Here's the drawing with two shaded views (mm, measured from the low corner). I have some questions. Round coordinates to 2 decimals unless told otherwise and drop trailing zeros. Order: outer loops, then holes, each group sorted by start corner. A loop starts at its lowest first (then second) coordinate and runs counter-clockwise, first axis right, second up.
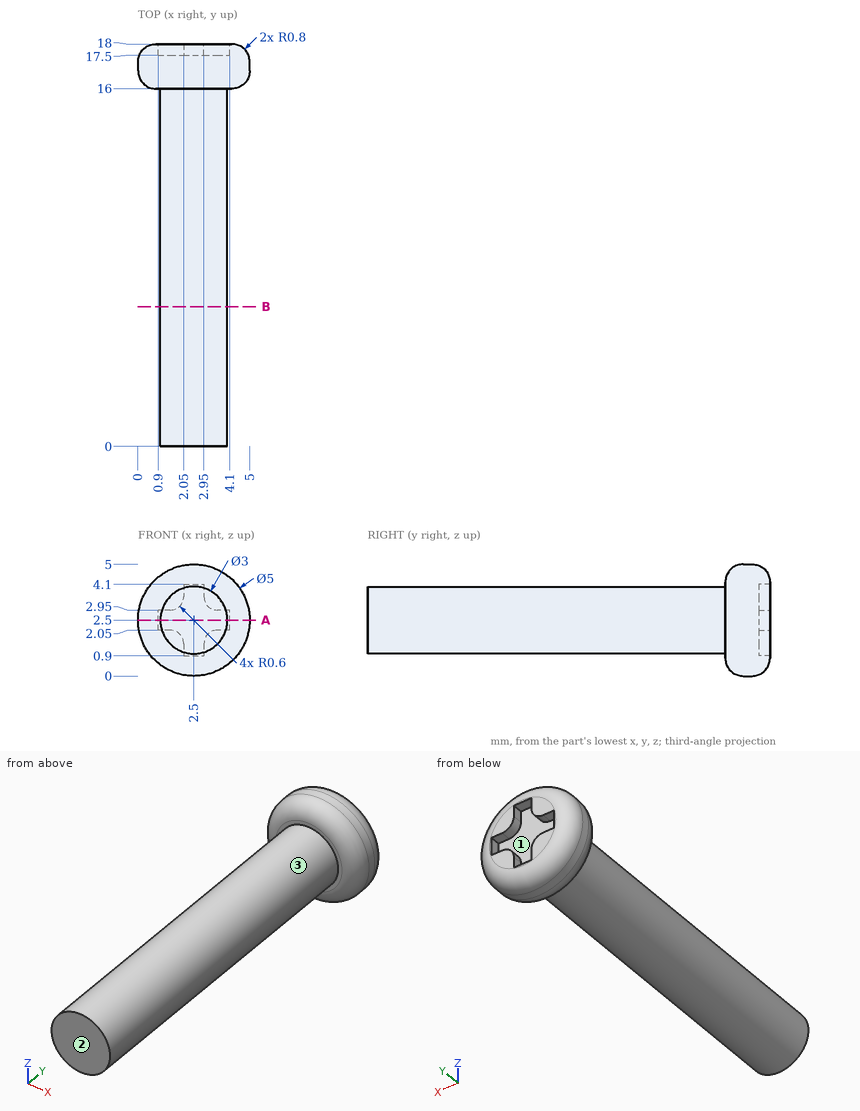
1. I need wall thicknesses on probe 1 along X at (y, z) = (13.5, 2.7); probe 2 along Z at (x, y) = (2.45, 4.75); probe 3 along Y at (x, z) = (2.75, 1.1). Which ranges of each line are inside material? Lowest first, please.
Evaluation:
probe 1: x = 1.01 to 3.99
probe 2: z = 1 to 4
probe 3: y = 0 to 17.5
2. I'm going to push flat-ended pins straight in: P1, Ø3, axis at y = 2.5, z = 2, coming from the +X side; P2, Ø1, axis at x = 3.5, y = 11.5, coming from the -Z side. Where does each tip first touch, or does it pass through?
Evaluation:
P1: stops at x = 4
P2: stops at z = 1.09
3. If we section it at A-A, the plane z = 2.5: Write out the boundary of the cut face in (x, y), and give its area (3 significant figures).
Evaluation:
outline: (0, 16.8) arc R0.8 ccw to (0.8, 16) - (1, 16) - (1, 0) - (4, 0) - (4, 16) - (4.2, 16) arc R0.8 ccw to (5, 16.8) - (5, 17.2) arc R0.8 ccw to (4.2, 18) - (4.1, 18) - (4.1, 17.5) - (0.9, 17.5) - (0.9, 18) - (0.8, 18) arc R0.8 ccw to (0, 17.2) - close
area: 55.9 mm2
4. If we section it at B-B, the plane y = 6.25: Write out the boundary of the cut face in (x, z).
Evaluation:
outline: circle Ø3 at (2.5, 2.5)
5. If we mould it in two halves opening along Z, with no side actions, what happens to the marked faces 1, 2 and 3? For each: released by +Z, released by -Z, zero draft, split by the parting line, or undercut.
Evaluation:
face 1: undercut
face 2: zero draft
face 3: split by the parting line
